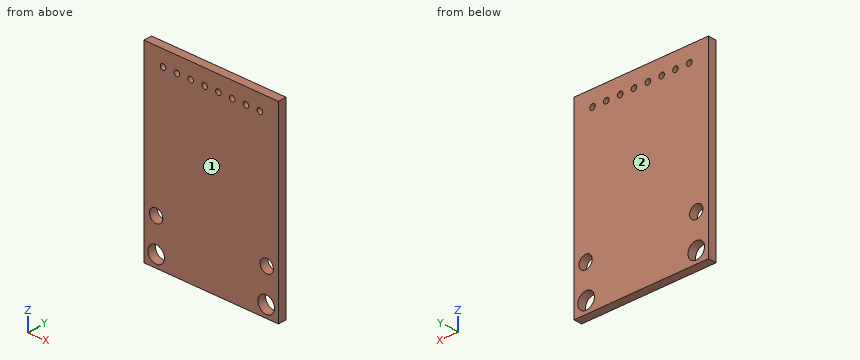
from build123d import *

# Parameters (mm, degrees)
SKETCH1_W             = 24.3
SKETCH1_H             = 34.1
BOSS_EXTRUDE1_DEPTH   = 1.5
F_3_0MM_DOWEL_HOLE1_D = 3
M2_CLEARANCE_HOLE1_D  = 2.4
CUT_EXTRUDE1_REACH    = 3.5
SKETCH9_R             = 0.5


with BuildPart() as part:
    # Sketch1 → Boss-Extrude1 (new body)
    with BuildSketch(Plane(origin=(0, 0, 0), x_dir=(1, 0, 0), z_dir=(0, 1, 0))):
        Rectangle(SKETCH1_W, SKETCH1_H)
    extrude(amount=BOSS_EXTRUDE1_DEPTH)

    # Ø3.0mm Dowel Hole1 (through all)
    with Locations(Plane(origin=(0, 1.5, 0), x_dir=(1, 0, 0), z_dir=(0, 1, 0))):
        with Locations((-9.95, 14.92), (9.95, 14.92)):
            Hole(F_3_0MM_DOWEL_HOLE1_D / 2)

    # M2 Clearance Hole1 (through all)
    with Locations(Plane(origin=(0, 1.5, 0), x_dir=(1, 0, 0), z_dir=(0, 1, 0))):
        with Locations((-9.95, 9), (10.05, 9)):
            Hole(M2_CLEARANCE_HOLE1_D / 2)

    # Sketch9 → Cut-Extrude1 (cut, up to next)
    with BuildSketch(Plane(origin=(0, 1.5, 0), x_dir=(1, 0, 0), z_dir=(0, 1, 0)), mode=Mode.PRIVATE) as cut_extrude1_sk1:
        with Locations((-8.7, -14.26)):
            Circle(SKETCH9_R)
    cut_extrude1_tool1 = extrude(cut_extrude1_sk1.sketch, amount=-CUT_EXTRUDE1_REACH, mode=Mode.PRIVATE) & part.part
    add(cut_extrude1_tool1.solids().sort_by_distance((-8.7, 1.5, 14.26))[0], mode=Mode.SUBTRACT)
    # Sketch9 → Cut-Extrude1 (cut, up to next)
    with BuildSketch(Plane(origin=(0, 1.5, 0), x_dir=(1, 0, 0), z_dir=(0, 1, 0)), mode=Mode.PRIVATE) as cut_extrude1_sk2:
        with Locations((-6.2, -14.26)):
            Circle(SKETCH9_R)
    cut_extrude1_tool2 = extrude(cut_extrude1_sk2.sketch, amount=-CUT_EXTRUDE1_REACH, mode=Mode.PRIVATE) & part.part
    add(cut_extrude1_tool2.solids().sort_by_distance((-6.2, 1.5, 14.26))[0], mode=Mode.SUBTRACT)
    # Sketch9 → Cut-Extrude1 (cut, up to next)
    with BuildSketch(Plane(origin=(0, 1.5, 0), x_dir=(1, 0, 0), z_dir=(0, 1, 0)), mode=Mode.PRIVATE) as cut_extrude1_sk3:
        with Locations((-3.7, -14.26)):
            Circle(SKETCH9_R)
    cut_extrude1_tool3 = extrude(cut_extrude1_sk3.sketch, amount=-CUT_EXTRUDE1_REACH, mode=Mode.PRIVATE) & part.part
    add(cut_extrude1_tool3.solids().sort_by_distance((-3.7, 1.5, 14.26))[0], mode=Mode.SUBTRACT)
    # Sketch9 → Cut-Extrude1 (cut, up to next)
    with BuildSketch(Plane(origin=(0, 1.5, 0), x_dir=(1, 0, 0), z_dir=(0, 1, 0)), mode=Mode.PRIVATE) as cut_extrude1_sk4:
        with Locations((-1.2, -14.26)):
            Circle(SKETCH9_R)
    cut_extrude1_tool4 = extrude(cut_extrude1_sk4.sketch, amount=-CUT_EXTRUDE1_REACH, mode=Mode.PRIVATE) & part.part
    add(cut_extrude1_tool4.solids().sort_by_distance((-1.2, 1.5, 14.26))[0], mode=Mode.SUBTRACT)
    # Sketch9 → Cut-Extrude1 (cut, up to next)
    with BuildSketch(Plane(origin=(0, 1.5, 0), x_dir=(1, 0, 0), z_dir=(0, 1, 0)), mode=Mode.PRIVATE) as cut_extrude1_sk5:
        with Locations((1.3, -14.26)):
            Circle(SKETCH9_R)
    cut_extrude1_tool5 = extrude(cut_extrude1_sk5.sketch, amount=-CUT_EXTRUDE1_REACH, mode=Mode.PRIVATE) & part.part
    add(cut_extrude1_tool5.solids().sort_by_distance((1.3, 1.5, 14.26))[0], mode=Mode.SUBTRACT)
    # Sketch9 → Cut-Extrude1 (cut, up to next)
    with BuildSketch(Plane(origin=(0, 1.5, 0), x_dir=(1, 0, 0), z_dir=(0, 1, 0)), mode=Mode.PRIVATE) as cut_extrude1_sk6:
        with Locations((3.8, -14.26)):
            Circle(SKETCH9_R)
    cut_extrude1_tool6 = extrude(cut_extrude1_sk6.sketch, amount=-CUT_EXTRUDE1_REACH, mode=Mode.PRIVATE) & part.part
    add(cut_extrude1_tool6.solids().sort_by_distance((3.8, 1.5, 14.26))[0], mode=Mode.SUBTRACT)
    # Sketch9 → Cut-Extrude1 (cut, up to next)
    with BuildSketch(Plane(origin=(0, 1.5, 0), x_dir=(1, 0, 0), z_dir=(0, 1, 0)), mode=Mode.PRIVATE) as cut_extrude1_sk7:
        with Locations((6.3, -14.26)):
            Circle(SKETCH9_R)
    cut_extrude1_tool7 = extrude(cut_extrude1_sk7.sketch, amount=-CUT_EXTRUDE1_REACH, mode=Mode.PRIVATE) & part.part
    add(cut_extrude1_tool7.solids().sort_by_distance((6.3, 1.5, 14.26))[0], mode=Mode.SUBTRACT)
    # Sketch9 → Cut-Extrude1 (cut, up to next)
    with BuildSketch(Plane(origin=(0, 1.5, 0), x_dir=(1, 0, 0), z_dir=(0, 1, 0)), mode=Mode.PRIVATE) as cut_extrude1_sk8:
        with Locations((8.8, -14.26)):
            Circle(SKETCH9_R)
    cut_extrude1_tool8 = extrude(cut_extrude1_sk8.sketch, amount=-CUT_EXTRUDE1_REACH, mode=Mode.PRIVATE) & part.part
    add(cut_extrude1_tool8.solids().sort_by_distance((8.8, 1.5, 14.26))[0], mode=Mode.SUBTRACT)


solid = part.part
Can you work these out from the model? Positions are in its coordinate system, mm. Face numbers are marked on the shaded views. Coordinates: 2 decimals unless noted, no trailing zeros. Write each loop counter-clockwise with the first axis right and the second up, starting at its lowest first coordinate (ties: lowest second). Pieces come first, ordered by that corner, then holes. Notation, with made-up numbers: (27.25, 25.25) -> (58.25, 25.25) arc R20 ccw to (58.25, 58.25) -> close; hole circle Ø9 at (-3.75, 74). An arc over 180 degrees is marked (long way). Write each question's results on one line, items separated by ' | '. Start each with the question number.
Q1. Imagine slicing it at D-D (x = 9.95). Write out the boundary of the cut face in (y, z), then the cut area to 3 significant figures.
Q2. We'd pull the mould along Y, two halves only. Please class the marked faces 1 and 2: +Y half, -Y half, draft (parallel to the pull), parting line (faces both ways), or undercut.
Q3. Imagine slicing it at C-C (z = -8.5). Write out the boundary of the cut face in (x, y), then the cut area to 3 significant figures.
Q4. Imagine slicing it at A-A (x = -1.2). Write out the boundary of the cut face in (y, z).
Q5. I'm going to push flat-ended pins straight in: pin 1 (4 mm diameter, centred on x = 9.95, z = -14.92, fed in from -Y); pin 2 (2.5 mm diameter, centred on x = -9.95, z = -14.92, fed in from -Y). Where does each tip first touch, or does it pass through?
Q6. If I drill on probe 1 along X at (y, z) = (1.1, -9); probe 2 along Z at (x, y) = (1.3, 0.9); probe 3 along Z at (x, y) = (-11, 0.45), over which ranges is the centre line in solid material (lowest first)?
Q7. Imagine slicing it at B-B (y = 0.6). State how many separate pieces and enclosed holes the cut face has, then the cut area to 3 significant figures.
Taken from the geometry:
1) outline: (0, -17.05) -> (1.5, -17.05) -> (1.5, -16.42) -> (0, -16.42) -> close; (0, -13.42) -> (1.5, -13.42) -> (1.5, -10.2) -> (0, -10.2) -> close; (0, -7.8) -> (1.5, -7.8) -> (1.5, 17.05) -> (0, 17.05) -> close | area: 43.1 mm^2
2) face 1: -Y half | face 2: +Y half
3) outline: (-12.15, 0) -> (-11.04, 0) -> (-11.04, 1.5) -> (-12.15, 1.5) -> close; (-8.86, 0) -> (8.96, 0) -> (8.96, 1.5) -> (-8.86, 1.5) -> close; (11.14, 0) -> (12.15, 0) -> (12.15, 1.5) -> (11.14, 1.5) -> close | area: 29.9 mm^2
4) outline: (0, -17.05) -> (1.5, -17.05) -> (1.5, 13.76) -> (0, 13.76) -> close; (0, 14.76) -> (1.5, 14.76) -> (1.5, 17.05) -> (0, 17.05) -> close
5) pin 1: stops at y = 0 | pin 2: passes through
6) probe 1: x = -12.15 to -11.15, -8.75 to 8.85, 11.25 to 12.15 | probe 2: z = -17.05 to 13.76, 14.76 to 17.05 | probe 3: z = -17.05 to -15.99, -13.85 to -9.58, -8.42 to 17.05
7) separate pieces: 1 | enclosed holes: 12 | area: 799 mm^2
